Check sheet for the modelled part. Datum: model origin and axes. Units: mm. Face numbers are marked on the shaded views. A direction names the side the tool comes from. Coordinates: 2 decimals unless noted, no trailing zeros. Write each loop counter-clockwise with the first axis right and the second up, starting at its lowest first coordinate (ties: lowest second). Pieces come first, ordered by that corner, then holes. Notation, with made-up numbers: (76, 36) -> (104, 36) arc R19 ccw to (104, 45) -> close; hole circle Ø7 at (16.25, -14). An arc over 180 degrees is marked (long way). One line per item, written item: value. Start each with the question number.
1) Sectioned sample at C-C on z = -24. Enter the section's corners in (x, y).
2) Set-up check for the marked faces 4, 5 and 6: record each of +Z, -Z, +X, -X, +Y, -Y from which the full face is reachable in a straight line by a thin tool's end or side.
3) Sectioned sample at B-B on x = 13.5. Enter the section's corners in (y, z), plus the area to 3 significant figures.
4) Scan lines: line 1 along Y through (x, z) = (30, 7); line 2 along Y through (x, z) = (-30.3, 0); line 3 along Y through (x, z) = (-20, 10). Record each from-to range of solid material in increasing order. Write a range as [from, to].
5) Gauge pin test, flat ends, axial feed: P1, Ø20, axis at x = -2.5, y = -39.5, coming from the +Z side; P2, Ø8, axis at y = 2, z = -25.5, coming from the +X side; P3, Ø5, axis at x = 26.5, y = 28, coming from the +Z side; P4, Ø2.5, axis at y = 48, z = 0, coming from the -X side. Record the tip position at first contact, or that the pin passes through.
6) Sectioned sample at A-A on y = 17.5. Enter the section's corners in (x, z), plus the area to 3 significant figures.
7) Draft check along Z on the marked faces 1, 2 and 3. Enter one of: +Z half, -Z half, draft (parallel to the pull), parting line (faces both ways), or undercut.
8) Sectioned sample at D-D on y = -39. Enter the section's corners in (x, z).
```python
from build123d import *

# Parameters (mm, degrees)
SKETCH1_W           = 63
SKETCH1_H           = 27
BOSS_EXTRUDE1_DEPTH = 60
SKETCH2_W           = 59
SKETCH2_H           = 27
CUT_EXTRUDE1_DEPTH  = 50
SKETCH3_R           = 1.5
CUT_EXTRUDE2_DEPTH  = 65
SKETCH5_W           = 20
SKETCH5_H           = 12
BOSS_EXTRUDE2_DEPTH = 30
SKETCH6_W           = 88
SKETCH6_H           = 32
BOSS_EXTRUDE3_DEPTH = 22
SKETCH7_W           = 83
SKETCH7_H           = 18
CUT_EXTRUDE3_DEPTH  = 30
SKETCH10_W          = 56
SKETCH10_H          = 20
CUT_EXTRUDE5_DEPTH  = 3
SKETCH11_W          = 23
SKETCH11_H          = 22
BOSS_EXTRUDE4_DEPTH = 1
SKETCH12_W          = 17
SKETCH12_H          = 18
CUT_EXTRUDE7_DEPTH  = 2.5
SKETCH13_W          = 31.74972829
SKETCH13_H          = 12
CUT_EXTRUDE9_DEPTH  = 2.5
CUT_EXTRUDE10_DEPTH = 2.5
SKETCH23_W          = 12
SKETCH23_H          = 10
BOSS_EXTRUDE7_DEPTH = 13
SKETCH25_R          = 3.5
CUT_EXTRUDE13_DEPTH = 13
SKETCH26_W          = 12
SKETCH26_H          = 10
BOSS_EXTRUDE8_DEPTH = 17
SKETCH27_R          = 3.5
CUT_EXTRUDE14_DEPTH = 17
SKETCH28_R          = 1
CUT_EXTRUDE15_DEPTH = 10


with BuildPart() as part:
    # Sketch1 → Boss-Extrude1 (new body)
    with BuildSketch(Plane(origin=(0, 0, 0), x_dir=(1, 0, 0), z_dir=(0, 1, 0))):
        Rectangle(SKETCH1_W, SKETCH1_H)
    extrude(amount=BOSS_EXTRUDE1_DEPTH)

    # Sketch2 → Cut-Extrude1 (cut)
    with BuildSketch(Plane(origin=(0, 60, 0), x_dir=(1, 0, 0), z_dir=(0, 1, 0))):
        Rectangle(SKETCH2_W, SKETCH2_H)
    extrude(amount=-CUT_EXTRUDE1_DEPTH, mode=Mode.SUBTRACT)

    # Sketch3 → Cut-Extrude2 (cut)
    with BuildSketch(Plane(origin=(31.5, 0, 0), x_dir=(0, 0, -1), z_dir=(1, 0, 0))):
        with Locations((0, 41)):
            Circle(SKETCH3_R)
    extrude(amount=-CUT_EXTRUDE2_DEPTH, mode=Mode.SUBTRACT)

    # Sketch5 → Boss-Extrude2 (add)
    with BuildSketch(Plane.XZ):
        with Locations((0, -7.5)):
            Rectangle(SKETCH5_W, SKETCH5_H)
    extrude(amount=BOSS_EXTRUDE2_DEPTH)

    # Sketch6 → Boss-Extrude3 (add)
    with BuildSketch(Plane.XZ.offset(30)):
        with Locations((0, -1.5)):
            Rectangle(SKETCH6_W, SKETCH6_H)
    extrude(amount=BOSS_EXTRUDE3_DEPTH)

    # Sketch7 → Cut-Extrude3 (cut)
    with BuildSketch(Plane.XY.offset(14.5)):
        with Locations((0.5, -41)):
            Rectangle(SKETCH7_W, SKETCH7_H)
    extrude(amount=-CUT_EXTRUDE3_DEPTH, mode=Mode.SUBTRACT)

    # Sketch10 → Cut-Extrude5 (cut)
    with BuildSketch(Plane.XZ.offset(52)):
        with Locations((0, -0.5)):
            Rectangle(SKETCH10_W, SKETCH10_H)
    extrude(amount=-CUT_EXTRUDE5_DEPTH, mode=Mode.SUBTRACT)

    # Sketch11 → Boss-Extrude4 (add)
    with BuildSketch(Plane.XY.offset(14.5)):
        with Locations((-32.5, -41)):
            Rectangle(SKETCH11_W, SKETCH11_H)
    extrude(amount=BOSS_EXTRUDE4_DEPTH)

    # Sketch12 → Cut-Extrude7 (cut)
    with BuildSketch(Plane(origin=(44, 0, 0), x_dir=(0, 0, -1), z_dir=(1, 0, 0))):
        with Locations((-6, -41)):
            Rectangle(SKETCH12_W, SKETCH12_H)
    extrude(amount=-CUT_EXTRUDE7_DEPTH, mode=Mode.SUBTRACT)

    # Sketch13 → Cut-Extrude9 (cut)
    with BuildSketch(Plane(origin=(0, -30, 0), x_dir=(1, 0, 0), z_dir=(0, 1, 0))):
        with Locations((-0.07313141, -8.5)):
            Rectangle(SKETCH13_W, SKETCH13_H)
    extrude(amount=-CUT_EXTRUDE9_DEPTH, mode=Mode.SUBTRACT)

    # Sketch16 → Cut-Extrude10 (cut)
    with BuildSketch(Plane(origin=(0, -30, 0), x_dir=(1, 0, 0), z_dir=(0, 1, 0))):
        Polygon((-21, -14.5), (-21, -2.38991446), (-15.947995555, -2.5), (-15.947995555, -14.5), align=None)
    extrude(amount=-CUT_EXTRUDE10_DEPTH, mode=Mode.SUBTRACT)

    # Sketch23 → Boss-Extrude7 (add)
    with BuildSketch(Plane(origin=(0, 0, -17.5), x_dir=(-1, 0, 0), z_dir=(0, 0, -1))):
        with Locations((0, -41)):
            Rectangle(SKETCH23_W, SKETCH23_H)
    extrude(amount=BOSS_EXTRUDE7_DEPTH)

    # Sketch25 → Cut-Extrude13 (cut)
    with BuildSketch(Plane(origin=(0, -36, 0), x_dir=(1, 0, 0), z_dir=(0, 1, 0))):
        with Locations(Location((0, 24, 0), (0, 0, 270))):
            Circle(SKETCH25_R)
    extrude(amount=-CUT_EXTRUDE13_DEPTH, mode=Mode.SUBTRACT)

    # Sketch26 → Boss-Extrude8 (add)
    with BuildSketch(Plane(origin=(0, 0, -13.5), x_dir=(-1, 0, 0), z_dir=(0, 0, -1))):
        Rectangle(SKETCH26_W, SKETCH26_H)
    extrude(amount=BOSS_EXTRUDE8_DEPTH)

    # Sketch27 → Cut-Extrude14 (cut)
    with BuildSketch(Plane(origin=(0, 5, 0), x_dir=(1, 0, 0), z_dir=(0, 1, 0))):
        with Locations(Location((0, 24, 0), (0, 0, 270))):
            Circle(SKETCH27_R)
    extrude(amount=-CUT_EXTRUDE14_DEPTH, mode=Mode.SUBTRACT)

    # Sketch28 → Cut-Extrude15 (cut)
    with BuildSketch(Plane(origin=(31.5, 0, 0), x_dir=(0, 0, -1), z_dir=(1, 0, 0))):
        with Locations((0, 48)):
            Circle(SKETCH28_R)
        with Locations((7, 41)):
            Circle(SKETCH28_R)
        with Locations((-7, 41)):
            Circle(SKETCH28_R)
    extrude(amount=-CUT_EXTRUDE15_DEPTH, mode=Mode.SUBTRACT)


solid = part.part
```
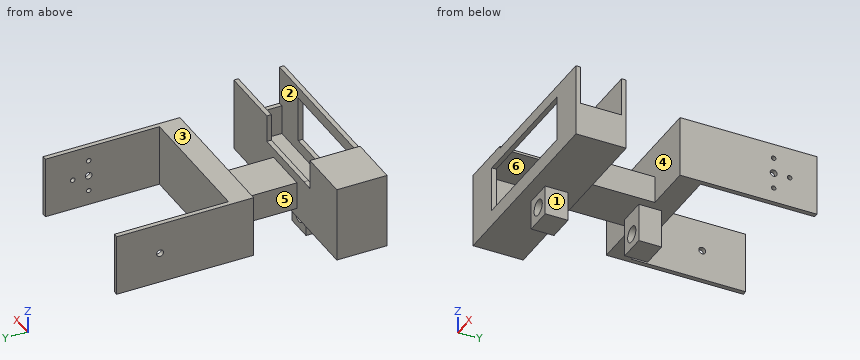
Answers:
1. outline: (-6, -46) -> (-3.5, -46) -> (-3.5, -36) -> (-6, -36) -> close; (-6, -5) -> (-3.5, -5) -> (-3.5, 5) -> (-6, 5) -> close; (3.5, -46) -> (6, -46) -> (6, -36) -> (3.5, -36) -> close; (3.5, -5) -> (6, -5) -> (6, 5) -> (3.5, 5) -> close
2. face 4: +Z
2. face 5: +Z, -Z, -X
2. face 6: +X
3. outline: (-52, -17.5) -> (-30, -17.5) -> (-30, 2.5) -> (-32, 2.5) -> (-32, -15.5) -> (-50, -15.5) -> (-50, -10.5) -> (-52, -10.5) -> close; (-52, 9.5) -> (-50, 9.5) -> (-50, 14.5) -> (-52, 14.5) -> close; (0, -13.5) -> (10, -13.5) -> (10, 13.5) -> (0, 13.5) -> close
3. area: 370 mm2
4. line 1: y = [-52, -50], [-32, -30], [0, 40], [42, 60]
4. line 2: y = [-52, -50], [-32, -30], [0, 39.5], [42.5, 60]
4. line 3: y = [-52, -50], [0, 10]
5. P1: stops at z = 2.5
5. P2: stops at x = 6
5. P3: passes through
5. P4: stops at x = -31.5
6. outline: (-31.5, -13.5) -> (-29.5, -13.5) -> (-29.5, 13.5) -> (-31.5, 13.5) -> close; (29.5, -13.5) -> (31.5, -13.5) -> (31.5, 13.5) -> (29.5, 13.5) -> close
6. area: 108 mm2
7. face 1: draft
7. face 2: undercut
7. face 3: +Z half
8. outline: (-44, -17.5) -> (-6, -17.5) -> (-6, -30.5) -> (6, -30.5) -> (6, -17.5) -> (44, -17.5) -> (44, -2.5) -> (42, -2.5) -> (42, -15.5) -> (-41, -15.5) -> (-41, 14.5) -> (-21, 14.5) -> (-21, 15.5) -> (-44, 15.5) -> close; hole circle Ø7 at (0, -24)
